Model file for the job. Use its own axes, mm. A direction names the side the tool comes from. Round coordinates to 2 decimals unless told otherwise and drop trailing zeros. Order: outer loops, then holes, each group sorted by start corner. A loop starts at its lowest first (then second) coordinate and runs counter-clockwise, first axis right, second up. Notation, with made-up numbers: (-6.75, -12.75) - (26.25, -12.75) arc R26 ccw to (26.25, 6.25) - close; hole circle Ø3 at (-33, 59.25). An arc over 180 degrees is marked (long way). Write item = value, one per line.
```python
from build123d import *

# Parameters (mm, degrees)
EXTRUDE_1_DEPTH     = 5
SKETCH_2_R          = 2.1
CUT_EXTRUDE_1_DEPTH = 6
FILLET_1_R          = 5
SKETCH_3_R          = 2.5
CUT_EXTRUDE_2_DEPTH = 6
SKETCH_4_R          = 2.1
CUT_EXTRUDE_3_DEPTH = 6
SKETCH_5_OUTSIDE_W  = 532.64
SKETCH_5_OUTSIDE_H  = 472.64
CUT_EXTRUDE_4_DEPTH = 6


with BuildPart() as part:
    # 草图1 → 凸台-拉伸1 (new body)
    with BuildSketch(Plane(origin=(0, 0, 0), x_dir=(1, 0, 0), z_dir=(0, 1, 0))):
        Polygon((-180, 180), (-180, 103), (-80, 103), (-80, 180), (80, 180), (80, 103), (180, 103), (180, 180), (210, 180), (210, -180), (180, -180), (180, -103), (80, -103), (80, -180), (-80, -180), (-80, -103), (-180, -103), (-180, -180), (-210, -180), (-210, 180), align=None)
    extrude(amount=EXTRUDE_1_DEPTH)

    # 草图2 → 切除-拉伸1 (cut, through all)
    with BuildSketch(Plane(origin=(0, 5, 0), x_dir=(1, 0, 0), z_dir=(0, 1, 0))):
        with Locations((115, -88.5)):
            Circle(SKETCH_2_R)
        with Locations((145, -88.5)):
            Circle(SKETCH_2_R)
        with Locations((130, -95.5)):
            Circle(SKETCH_2_R)
        with Locations((130, 95.5)):
            Circle(SKETCH_2_R)
        with Locations((145, 88.5)):
            Circle(SKETCH_2_R)
        with Locations((115, 88.5)):
            Circle(SKETCH_2_R)
        with Locations((-115, 88.5)):
            Circle(SKETCH_2_R)
        with Locations((-145, 88.5)):
            Circle(SKETCH_2_R)
        with Locations((-130, 95.5)):
            Circle(SKETCH_2_R)
        with Locations((-130, -95.5)):
            Circle(SKETCH_2_R)
        with Locations((-145, -88.5)):
            Circle(SKETCH_2_R)
        with Locations((-115, -88.5)):
            Circle(SKETCH_2_R)
    extrude(amount=-CUT_EXTRUDE_1_DEPTH, mode=Mode.SUBTRACT)

    # 圆角1
    fillet_1_edges = [part.edges().sort_by_distance(p)[0] for p in [
        (180, 2.5, 180),
        (80, 2.5, 180),
        (-80, 2.5, 180),
        (-180, 2.5, 180),
        (-180, 2.5, -180),
        (-80, 2.5, -180),
        (80, 2.5, -180),
        (180, 2.5, -180),
    ]]
    fillet(fillet_1_edges, radius=FILLET_1_R)

    # 草图3 → 切除-拉伸2 (cut, through all)
    with BuildSketch(Plane.XZ):
        with Locations((84.75, 31.75)):
            Circle(SKETCH_3_R)
        with Locations((84.75, -31.75)):
            Circle(SKETCH_3_R)
        with Locations((171.25, 31.75)):
            Circle(SKETCH_3_R)
        with Locations((171.25, -31.75)):
            Circle(SKETCH_3_R)
        with Locations((-171.25, -31.75)):
            Circle(SKETCH_3_R)
        with Locations((-171.25, 31.75)):
            Circle(SKETCH_3_R)
        with Locations((-84.75, -31.75)):
            Circle(SKETCH_3_R)
        with Locations((-84.75, 31.75)):
            Circle(SKETCH_3_R)
    extrude(amount=-CUT_EXTRUDE_2_DEPTH, mode=Mode.SUBTRACT)

    # 草图4 → 切除-拉伸3 (cut, through all)
    with BuildSketch(Plane.XZ):
        with Locations((-125, 0)):
            Circle(SKETCH_4_R)
        with Locations((125, 0)):
            Circle(SKETCH_4_R)
        with Locations((0, 10)):
            Circle(SKETCH_4_R)
        with Locations((0, -10)):
            Circle(SKETCH_4_R)
    extrude(amount=-CUT_EXTRUDE_3_DEPTH, mode=Mode.SUBTRACT)

    # 草图5 outside → 切除-拉伸4 (cut, through all)
    with BuildSketch(Plane.XZ):
        Rectangle(SKETCH_5_OUTSIDE_W, SKETCH_5_OUTSIDE_H)
        Polygon((-150, 16), (-150, -16), (-30, -16), (-30, -37), (30, -37), (30, -16), (150, -16), (150, 16), (30, 16), (30, 37), (-30, 37), (-30, 16), align=None, mode=Mode.SUBTRACT)
    extrude(amount=-CUT_EXTRUDE_4_DEPTH, mode=Mode.SUBTRACT)


solid = part.part
```
1) 3-axis set-ups, long thin cutter, end or side, ignore diameter. For faces 1 (the face through (91, 2, 16)), 2 (the face through (89, 2, -16)), 3 (the face through (-91, 2, -16)), 4 (the face through (-89, 2, 16)): which of +Z, -Z, +X, -X, +Y, -Y reach the whole face in a straight line?
Conclusion:
face_1 = +Z, +X, +Y, -Y
face_2 = -Z, +X, +Y, -Y
face_3 = -Z, -X, +Y, -Y
face_4 = +Z, -X, +Y, -Y
2) Cut at B-B (z = -28.5). Write the cut outline in (x, y), and give its area (3 significant figures).
Conclusion:
outline = (-30, 0) - (30, 0) - (30, 5) - (-30, 5) - close
area = 300 mm^2
3) Cut at A-A (y = 3.9). Write the cut outline in (x, z), and give its area (3 significant figures).
Conclusion:
outline = (-150, -16) - (-30, -16) - (-30, -37) - (30, -37) - (30, -16) - (150, -16) - (150, 16) - (30, 16) - (30, 37) - (-30, 37) - (-30, 16) - (-150, 16) - close; hole circle Ø4.2 at (-125, 0); hole circle Ø4.2 at (0, -10); hole circle Ø4.2 at (0, 10); hole circle Ø4.2 at (125, 0)
area = 12,100 mm^2
4) Wall check: line 1 along Z through (x, y) = (0, 1.6); line 2 along X through (y, z) = (3.75, 18); line 3 along Z through (x, y) = (49, 4.55). Give the ranges that are in metal, low to high.
Conclusion:
line_1 = -37 to -12.1, -7.9 to 7.9, 12.1 to 37
line_2 = -30 to 30
line_3 = -16 to 16
5) Cut at C-C (x = -67.5). Write the cut outline in (y, z).
Conclusion:
outline = (0, -16) - (5, -16) - (5, 16) - (0, 16) - close
6) Flat gauge pins, fed straight in: pin 1 Ø3 at (x, y) = (54, 1.5) entering from +Z; pin 2 Ø2.5 at (x, y) = (110.5, 3) entering from -Z; pin 3 Ø4 at (x, z) = (0, 10) entering from +Y; pin 4 Ø6.5 at (x, z) = (-125, 0) entering from +Y. Where does each tip first touch, or does it go through?
Conclusion:
pin_1 = 16
pin_2 = -16
pin_3 = through
pin_4 = 5
